```python
from build123d import *

# Parameters (mm, degrees)
SKETCH1_W           = 98
SKETCH1_H           = 98
BOSS_EXTRUDE2_DEPTH = 5
SKETCH6_R           = 2.5
SKETCH6_R_2         = 2.516988407
CUT_EXTRUDE11_DEPTH = 19
SKETCH9_R           = 12.25
CUT_EXTRUDE10_DEPTH = 19
SKETCH10_W          = 35
SKETCH10_H          = 40
SKETCH10_W_2        = 32
SKETCH10_H_2        = 37
CUT_EXTRUDE12_DEPTH = 1
SKETCH12_W          = 88
SKETCH12_H          = 88
SKETCH12_W_2        = 78
SKETCH12_H_2        = 78
BOSS_EXTRUDE4_DEPTH = 2
SKETCH13_R          = 1.75
CUT_EXTRUDE13_DEPTH = 2
SKETCH14_R          = 1
CUT_EXTRUDE14_DEPTH = 9


with BuildPart() as part:
    # Sketch1 → Boss-Extrude2 (new body)
    with BuildSketch(Plane(origin=(0, 0, 0), x_dir=(1, 0, 0), z_dir=(0, 1, 0))):
        Rectangle(SKETCH1_W, SKETCH1_H)
    extrude(amount=BOSS_EXTRUDE2_DEPTH)

    # Sketch6 → Cut-Extrude11 (cut)
    with BuildSketch(Plane(origin=(0, 5, 0), x_dir=(1, 0, 0), z_dir=(0, 1, 0))):
        with Locations(Location((-12.5, 36.5, 0), (0, 0, 270))):
            Circle(SKETCH6_R)
        with Locations(Location((12.5, 36.5, 0), (0, 0, 270))):
            Circle(SKETCH6_R)
        with Locations(Location((-12.5, 6.5, 0), (0, 0, 270))):
            Circle(SKETCH6_R)
        with Locations(Location((12.5, 6.5, 0), (0, 0, 270))):
            Circle(SKETCH6_R)
        with Locations(Location((-31.5, -6.5, 0), (0, 0, 270))):
            Circle(SKETCH6_R_2)
        with Locations(Location((-6.5, -6.5, 0), (0, 0, 270))):
            Circle(SKETCH6_R)
        with Locations(Location((-31.5, -36.5, 0), (0, 0, 270))):
            Circle(SKETCH6_R)
        with Locations(Location((-6.5, -36.5, 0), (0, 0, 270))):
            Circle(SKETCH6_R)
        with Locations(Location((6.5, -36.5, 0), (0, 0, 270))):
            Circle(SKETCH6_R)
        with Locations(Location((31.5, -36.5, 0), (0, 0, 270))):
            Circle(SKETCH6_R)
        with Locations(Location((6.5, -6.5, 0), (0, 0, 270))):
            Circle(SKETCH6_R)
        with Locations(Location((31.5, -6.5, 0), (0, 0, 270))):
            Circle(SKETCH6_R_2)
    extrude(amount=-CUT_EXTRUDE11_DEPTH, mode=Mode.SUBTRACT)

    # Sketch9 → Cut-Extrude10 (cut)
    with BuildSketch(Plane.XZ):
        with Locations(Location((0, -20.5, 0), (0, 0, 270))):
            Circle(SKETCH9_R)
        with Locations(Location((19, 20.5, 0), (0, 0, 270))):
            Circle(SKETCH9_R)
        with Locations(Location((-19, 20.5, 0), (0, 0, 270))):
            Circle(SKETCH9_R)
    extrude(amount=-CUT_EXTRUDE10_DEPTH, mode=Mode.SUBTRACT)

    # Sketch10 → Cut-Extrude12 (cut)
    # profile 1 of 3: a face of its own
    with BuildSketch(Plane(origin=(0, 5, 0), x_dir=(1, 0, 0), z_dir=(0, 1, 0))):
        with Locations((0, 21.5)):
            Rectangle(SKETCH10_W, SKETCH10_H)
        with Locations((0, 21.5)):
            Rectangle(SKETCH10_W_2, SKETCH10_H_2, mode=Mode.SUBTRACT)
    # profile 2 of 3: a face of its own
    with BuildSketch(Plane(origin=(0, 5, 0), x_dir=(1, 0, 0), z_dir=(0, 1, 0))):
        with Locations((-19, -21.5)):
            Rectangle(SKETCH10_W, SKETCH10_H)
        with Locations((-19, -21.5)):
            Rectangle(SKETCH10_W_2, SKETCH10_H_2, mode=Mode.SUBTRACT)
    # profile 3 of 3: a face of its own
    with BuildSketch(Plane(origin=(0, 5, 0), x_dir=(1, 0, 0), z_dir=(0, 1, 0))):
        with Locations((19, -21.5)):
            Rectangle(SKETCH10_W, SKETCH10_H)
        with Locations((19, -21.5)):
            Rectangle(SKETCH10_W_2, SKETCH10_H_2, mode=Mode.SUBTRACT)
    extrude(amount=-CUT_EXTRUDE12_DEPTH, mode=Mode.SUBTRACT)

    # Sketch12 → Boss-Extrude4 (add)
    with BuildSketch(Plane.XZ):
        Rectangle(SKETCH12_W, SKETCH12_H)
        Rectangle(SKETCH12_W_2, SKETCH12_H_2, mode=Mode.SUBTRACT)
    extrude(amount=BOSS_EXTRUDE4_DEPTH)

    # Sketch13 → Cut-Extrude13 (cut)
    with BuildSketch(Plane(origin=(0, 5, 0), x_dir=(1, 0, 0), z_dir=(0, 1, 0))):
        with BuildLine():
            ThreePointArc((0, -44.75), (-1.75, -46.5), (0, -48.25))
            Line((0, -48.25), (0, -44.75))
        make_face()
        with BuildLine():
            Line((0, -44.75), (0, -48.25))
            ThreePointArc((0, -48.25), (1.237436867, -47.737436867), (1.75, -46.5))
            ThreePointArc((1.75, -46.5), (1.237436867, -45.262563133), (0, -44.75))
        make_face()
        with Locations(Location((-46.5, 0, 0), (0, 0, 270))):
            Circle(SKETCH13_R)
        with Locations(Location((0, 46.5, 0), (0, 0, 270))):
            Circle(SKETCH13_R)
        with BuildLine():
            ThreePointArc((44.75, 0), (46.5, -1.75), (48.25, 0))
            Line((48.25, 0), (44.75, 0))
        make_face()
        with BuildLine():
            Line((44.75, 0), (48.25, 0))
            ThreePointArc((48.25, 0), (46.5, 1.75), (44.75, 0))
        make_face()
    extrude(amount=-CUT_EXTRUDE13_DEPTH, mode=Mode.SUBTRACT)

    # Sketch14 → Cut-Extrude14 (cut)
    with BuildSketch(Plane(origin=(0, 5, 0), x_dir=(1, 0, 0), z_dir=(0, 1, 0))):
        with Locations(Location((0, -46.5, 0), (0, 0, 270))):
            Circle(SKETCH14_R)
        with Locations(Location((-46.5, 0, 0), (0, 0, 270))):
            Circle(SKETCH14_R)
        with Locations(Location((46.5, 0, 0), (0, 0, 270))):
            Circle(SKETCH14_R)
        with Locations(Location((0, 46.5, 0), (0, 0, 270))):
            Circle(SKETCH14_R)
    extrude(amount=-CUT_EXTRUDE14_DEPTH, mode=Mode.SUBTRACT)


solid = part.part
```
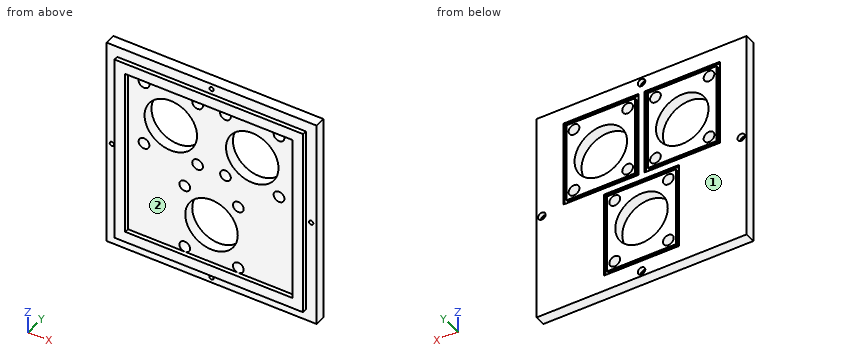
Geometry: final body of the model. Coordinates: model frame, mm. Face numbers are marked on the shaded views. Give positions to 0.01 mm unless a question says otherwise; leave off trailing zeros. Order: outer loops, then holes, each group sorted by start corner. A loop starts at its lowest first (then second) coordinate and runs counter-clockwise, first axis right, second up. Notation, with made-up numbers: M 36,5.5 L 43,5.5 A22 cw 43,12.5 Z; hole C 18.25,-17.5 d5. An arc over 180 degrees is marked long. Answer as CSV lines item,"result". Start each with the question number.
1) Mould query, pull axis X, two halves, no side actions, for the marked faces 1 and 2. Classes: +X half, -X half, draft (parallel to the pull), parting line (faces both ways), or undercut.
2) Cut plane D-D (x = -41). Output: boundary loops of the cut face in (y, z), then the cut area to 3 significant figures.
3) First-contact query: P1, Ø4, axis at x = -12.5, z = -6.5, coming from the +Y side; P2, Ø2.5, axis at x = 46.5, z = 0, coming from the -Y side; P3, Ø1.6, axis at x = -2.5, y = -1, coming from the +Z side; P4, Ø2.5, axis at x = -46.5, z = 0, coming from the +Y side. Flat tips, straight axial feed; report the tip coordinate or a pass-through.
4) Line query: line 1 (X direction, y = 3.8, z = 36.5); line 2 (X direction, y = 4, z = 0); line 3 (X direction, y = 2, z = 29.5). Output: solid intervals per line, ascending. Write a range as from..to.
5) Cut plane C-C (y = 1.5). State how many separate pieces and enclosed holes the cut face has, then the cut area to 3 significant figures.
6) Cut plane A-A (x = -19). Output: boundary loops of the cut face in (y, z), then the cut area to 4 significant figures.
7) Cut plane B-B (z = -20.5). Output: boundary loops of the cut face in (x, y).
Findings below:
1,face 1,"draft"
1,face 2,"undercut"
2,outline,"M -2,-44 L 0,-44 L 0,-49 L 5,-49 L 5,49 L 0,49 L 0,44 L -2,44 Z"
2,area,"666 mm²"
3,P1,"passes through"
3,P2,"stops at y = 0"
3,P3,"stops at z = 44"
3,P4,"stops at y = 3"
4,line 1,"x = -49..-34, -29..-9, -4..4, 9..29, 34..49"
4,line 2,"x = -49..-48.25, -44.75..44.75, 48.25..49"
4,line 3,"x = -49..-27.31, -10.69..10.69, 27.31..49"
5,separate pieces,"1"
5,enclosed holes,"19"
5,area,"7,940 mm²"
6,outline,"M -2,-44 L 0,-44 L 0,-49 L 5,-49 L 5,1.5 L 4,1.5 L 4,3 L 5,3 L 5,8.25 L 0,8.25 L 0,-39 L -2,-39 Z; M -2,39 L 0,39 L 0,32.75 L 5,32.75 L 5,40 L 4,40 L 4,41.5 L 5,41.5 L 5,49 L 0,49 L 0,44 L -2,44 Z"
6,area,"384.5 mm²"
7,outline,"M -49,0 L -44,0 L -44,-2 L -39,-2 L -39,0 L -12.25,0 L -12.25,5 L -16,5 L -16,4 L -17.5,4 L -17.5,5 L -49,5 Z; M 12.25,0 L 39,0 L 39,-2 L 44,-2 L 44,0 L 49,0 L 49,5 L 17.5,5 L 17.5,4 L 16,4 L 16,5 L 12.25,5 Z"
